Geometry: see drawing. Coordinates: mm, zero at the bounding-box minimum. Give positions to 0.01 mm unless a question says otherwise; leave off trailing zeros. Loops run counter-clockwise (first coordinate to the right, second up) from the corner with the lowest first, then second, coordinate; pieces in that order, holes last. Notation, with made-up numbers: (19.25, 59) -> (36.25, 59) arc R21 cw to (36.25, 75) -> close; hole circle Ø1 at (-24, 46.5). An arc over 180 degrees is marked (long way). One line per question, with ' | ' between items.
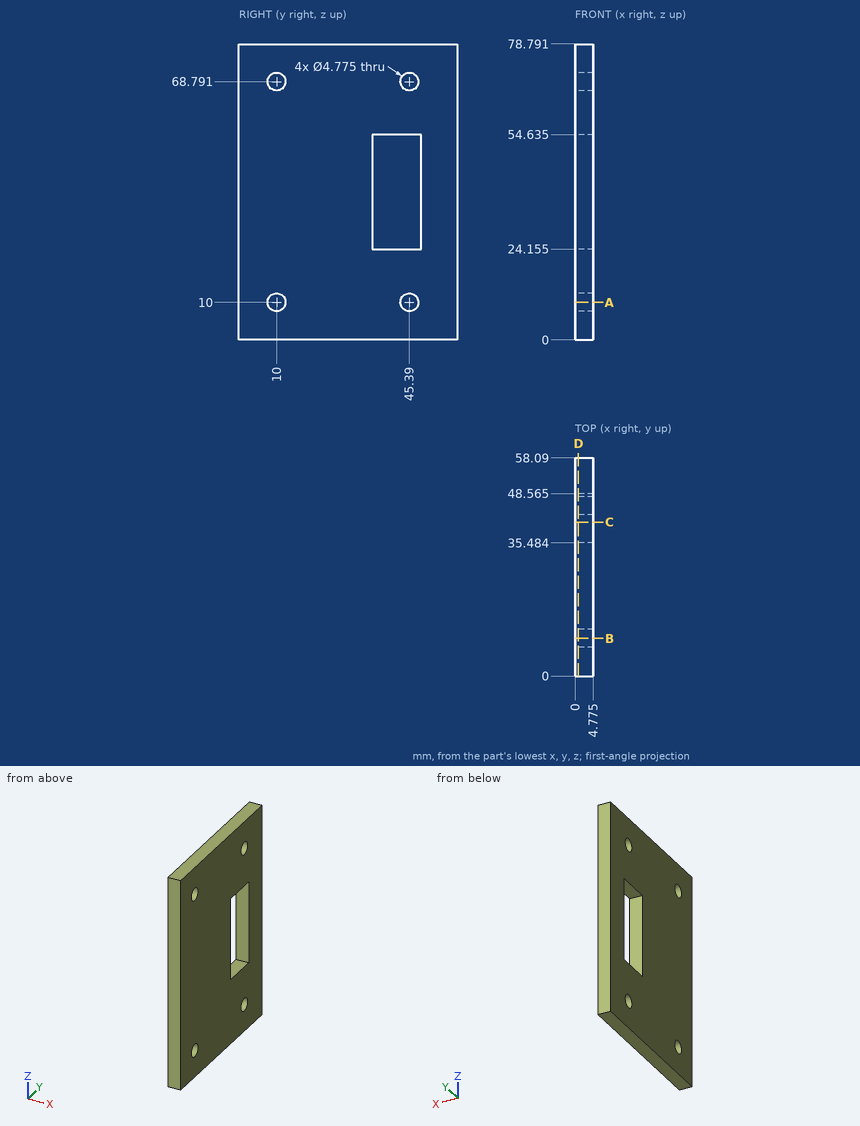
1. Section query B-B (y = 10). Output: boundary loops of the cut face in (x, z) (1 decimal), then the cut area to 3 significant figures.
Determined:
outline: (0, 0) -> (4.8, 0) -> (4.8, 7.6) -> (0, 7.6) -> close; (0, 12.4) -> (4.8, 12.4) -> (4.8, 66.4) -> (0, 66.4) -> close; (0, 71.2) -> (4.8, 71.2) -> (4.8, 78.8) -> (0, 78.8) -> close | area: 331 mm2
2. Pin query (flat end, axial travel): P1, Ø6, axis at y = 10, z = 68.79, coming from the -X side; P2, Ø3, axis at y = 10, z = 10, coming from the +X side. Return the tip coordinate at first contact, or that it passes through.
Determined:
P1: stops at x = 0 | P2: passes through
3. Section query A-A (z = 10). Output: boundary loops of the cut face in (x, y) (1 decimal), then the cut area to 3 significant figures.
Determined:
outline: (0, 0) -> (4.8, 0) -> (4.8, 7.6) -> (0, 7.6) -> close; (0, 12.4) -> (4.8, 12.4) -> (4.8, 43) -> (0, 43) -> close; (0, 47.8) -> (4.8, 47.8) -> (4.8, 58.1) -> (0, 58.1) -> close | area: 232 mm2
4. Ray query, line 1 along Y through (x, z) = (3.25, 10); line 2 along Y through (x, z) = (0.2, 49.5) (1 decimal); line 3 along Z through (x, y) = (1.15, 10). Return the intervals inside material, ascending. Write a range as from..to.
Determined:
line 1: y = 0..7.61, 12.39..43, 47.78..58.09 | line 2: y = 0..35.5, 48.6..58.1 | line 3: z = 0..7.61, 12.39..66.4, 71.18..78.79
5. Section query D-D (x = 0.9). Output: boundary loops of the cut face in (y, z) (1 decimal).
Determined:
outline: (0, 0) -> (58.1, 0) -> (58.1, 78.8) -> (0, 78.8) -> close; hole circle Ø4.8 at (10, 10); hole circle Ø4.8 at (10, 68.8); hole (35.5, 24.2) -> (48.6, 24.2) -> (48.6, 54.6) -> (35.5, 54.6) -> close; hole circle Ø4.8 at (45.4, 10); hole circle Ø4.8 at (45.4, 68.8)
6. Section query C-C (y = 41). Output: boundary loops of the cut face in (x, z) (1 decimal).
Determined:
outline: (0, 0) -> (4.8, 0) -> (4.8, 24.2) -> (0, 24.2) -> close; (0, 54.6) -> (4.8, 54.6) -> (4.8, 78.8) -> (0, 78.8) -> close
